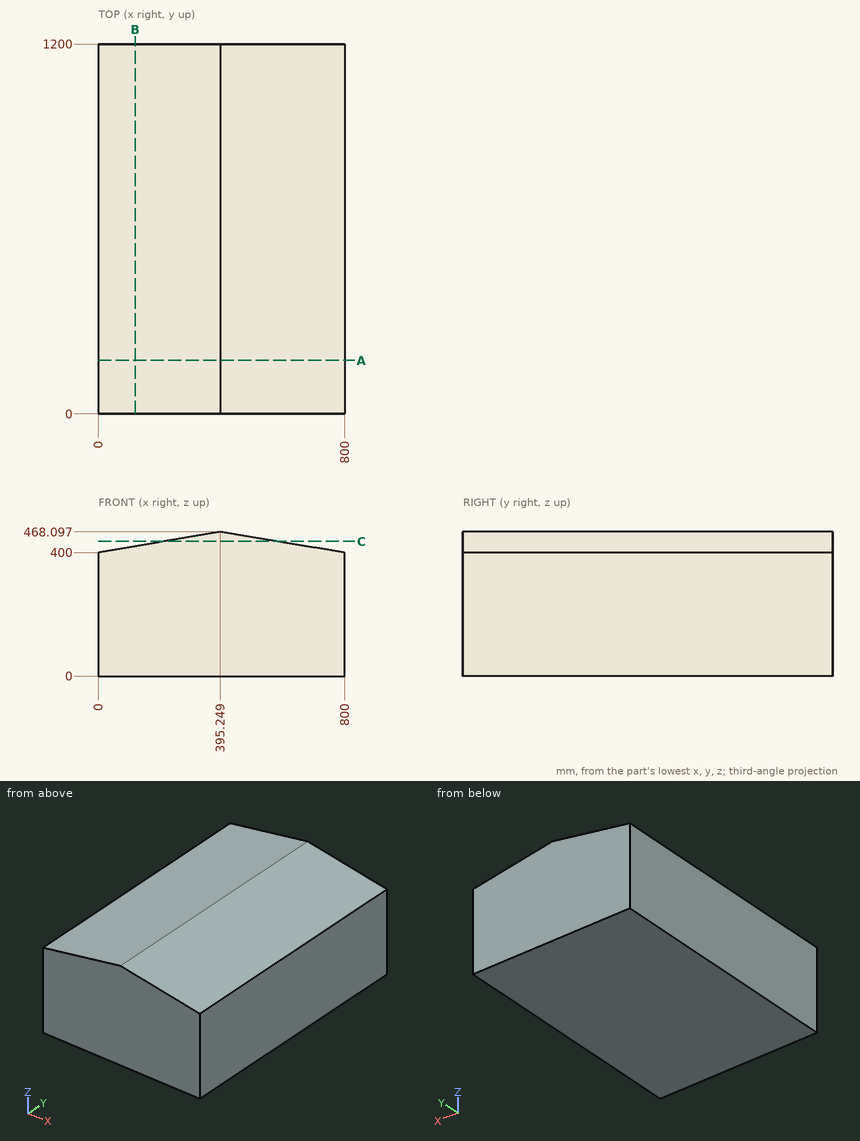
Job drawing, mm, ordinate dimensions from the low corner. One solid piece. Give positions to 0.01 mm unless a question says otherwise; leave off trailing zeros. Loops run counter-clockwise (first coordinate to the right, second up) from the corner with the lowest first, then second, coordinate; pieces in that order, holes last. Notation, with made-up numbers: M -2,14.5 L 22,14.5 A33 ccw 22,51.5 Z; hole C -4,47.5 d11. An arc over 180 degrees is marked long. Return JSON: item names as keys, results as strings.
1) Saw through at C-C, the plane z = 437. List the corners of the cut face in (x, y) (1 decimal), then the cut area to 3 significant figures.
Calculated:
{"outline": "M 214.8,0 L 580.1,0 L 580.1,1200 L 214.8,1200 Z", "area": "438,000 mm2"}
2) Drill centre lines: line 1 (Z direction, x = 622, y = 1019); line 2 (Z direction, x = 755, y = 57). Where is each one in solid material? Low to high.
Calculated:
{"line 1": "z = 0 to 429.95", "line 2": "z = 0 to 407.57"}
3) Saw through at A-A, the plane y = 173. List the corners of the cut face in (x, z), then the cut area to 3 significant figures.
Calculated:
{"outline": "M 0,0 L 800,0 L 800,400 L 395.25,468.1 L 0,400 Z", "area": "347,000 mm2"}
4) Flat gauge pin, fed straight in: pin 1 Ø2 at (x, y) = (201.5, 942.5) entering from +Z. Where does the tip first touch, or does it go through?
Calculated:
{"pin 1": "stops at z = 434.89"}
5) Saw through at B-B, the plane x = 119.5. List the corners of the cut face in (y, z), then the cut area to 3 significant figures.
Calculated:
{"outline": "M 0,0 L 1200,0 L 1200,420.59 L 0,420.59 Z", "area": "505,000 mm2"}
